Design review of the part built by this model. Coordinates are the model's own, in mm. Face numbers are marked on the shaded views. A direction names the side the tool comes from. Coordinates: 2 decimals unless noted, no trailing zeros. Write each loop counter-clockwise with the first axis right and the second up, starting at its lowest first coordinate (ties: lowest second). Pieces come first, ordered by that corner, then holes.
Q1. Add section C-C, the plane x = 40. Give the boundary of the cut face in (y, z).
Q2. Add section A-A, the plane y = 24. Give the boundary of the cut face in (x, z) (3 decimals), plus the area to 3 significant figures.
Q3. To check wall thickness, follow probe 1 along X at (y, z) = (157, -73); probe 2 along Z at (x, y) = (-6.5, 123.5); probe 3 along Z at (x, y) = (54, 81.5). State the ranges of each line that lie inside material, in increasing order.
Q4. Machinability: for the marked faces 4, 5 and 6, which of the approach directions +Z, -Z, +X, -X, +Y, -Y give a long, thin tool a straight path to every point of the face, cutting with its end or side? Answer none if there is none.
Q5. Clearance check with flat-ended pins moving along their axes: pin 1 Ø9.5 at (y, z) = (230, -51) entering from -X (3 decimals); pin 2 Ø2 at (x, z) = (218, 40.5) entering from +Y; pin 3 Ø15 at (x, y) = (-10, 100) entering from -Z. State where each tip first meets the part, or that it passes through.
Q6. Add section B-B, the plane z = -71. Give the boundary of the cut face in (x, y) (3 decimals).
Q7. Add section D-D, the plane y = 218. Give the boundary of the cut face in (x, z) (3 decimals).
Q8. The part is to be moulded in two halves that separate along Y. For the marked faces 1, 2 and 3, say which applies: +Y half, -Y half, draft (parallel to the pull), parting line (faces both ways), or undercut.
Autodesk Inventor part; units mm, degrees
ref_plane "Work Plane1" through (0, 104.775, 0) normal (0, 1, 0) x (-1, 0, 0)
ref_plane "Work Plane2" through (295.275, 0, -196.85) normal (-1, 0, 0) x (0, 0, 1)
ref_plane "YZ Plane" through (0, 0, 0) normal (1, 0, 0) x (0, 1, 0)
sketch "Sketch1" plane through (0, 0, 0) normal (1, 0, 0) x (0, 1, 0)
  line L0 (0, 120.65) -> (184.15, 120.65)
  line L1 (184.15, 120.65) -> (184.15, -120.65)
  line L2 (184.15, -120.65) -> (0, -120.65)
  line L3 (0, -120.65) -> (0, 120.65)
  point P0 (0, 0)
  point P1 (0, 0)
  dimension "d0" = 184.15
  dimension "d1" = 241.3
extrude "Extrusion1" add sketch "Sketch1" along normal blind 295.275
sketch "Sketch2" plane through (0, 0, 0) normal (-1, 0, 0) x (0, 0, 1)
  line L0 (120.65, 0) -> (120.65, 184.15) construction
  line L1 (120.65, 184.15) -> (-120.65, 184.15) construction
  line L2 (-120.65, 184.15) -> (-120.65, 0) construction
  line L3 (-120.65, 0) -> (120.65, 0) construction
  line L4 (-107.95, 171.45) -> (107.95, 171.45)
  line L5 (107.95, 171.45) -> (107.95, 12.7)
  line L6 (107.95, 12.7) -> (-107.95, 12.7)
  line L7 (-107.95, 12.7) -> (-107.95, 171.45)
  point P0 (0, 0)
  dimension "d4" = 12.7
extrude "Extrusion2" add sketch "Sketch2" along normal blind 19.05
ref_plane "Work Plane1" through (0, 104.775, 0) normal (0, 1, 0) x (-1, 0, 0)
sketch "Sketch3" plane through (0, 104.775, 0) normal (0, 1, 0) x (-1, 0, 0)
  line L0 (0, 120.65) -> (0, -120.65) construction
  line L1 (133.2378, 0) -> (-22.2063, 0) construction
  line L2 (0, 0) -> (19.05, 0)
  arc A0 (19.05, 0) -> (95.25, 76.2) centre (19.05, 76.2) ccw
  dimension "d8" = 19.05
  dimension "d22" = 76.2
sketch "Sketch4" plane through (0, 0, 0) normal (-1, 0, 0) x (0, 0, 1)
  circle A0 centre (0, 104.775) radius 9.525
  point P0 (0, 0)
  dimension "d9" = 19.05
sweep "Sweep1" add profiles "Sketch4" path "Sketch3"
sketch "Sketch5" plane through (0, 0, 0) normal (0, 1, 0) x (-1, 0, 0)
  line L0 (-295.275, 120.65) -> (-295.275, -120.65) construction
  line L1 (-295.275, 57.15) -> (-666.75, 57.15)
  line L2 (-666.75, 57.15) -> (-666.75, -196.85)
  line L3 (-666.75, -196.85) -> (-295.275, -196.85)
  line L4 (-295.275, -196.85) -> (-295.275, 57.15)
  line L5 (0, -120.65) -> (0, 120.65) construction
  point P0 (0, 0)
  dimension "d12" = 666.75
  dimension "d13" = 76.2
  dimension "d14" = 254
extrude "Extrusion3" add sketch "Sketch5" along normal blind 355.6
sketch "Sketch6" plane through (0, 0, 0) normal (0, 1, 0) x (-1, 0, 0)
  line L0 (-168.275, -63.5) -> (-295.275, -63.5)
  line L1 (-295.275, -63.5) -> (-295.275, -44.45)
  line L2 (-295.275, -44.45) -> (-168.275, -44.45)
  line L3 (-168.275, -44.45) -> (-168.275, -63.5)
  line L4 (-295.275, -196.85) -> (-295.275, 57.15) construction
  line L5 (0, -120.65) -> (-295.275, -120.65) construction
  point P0 (0, 0)
  dimension "d17" = 127
  dimension "d18" = 19.05
  dimension "d19" = 57.15
extrude "Extrusion4" add sketch "Sketch6" along normal blind 247.65
ref_plane "Work Plane2" through (295.275, 0, -196.85) normal (-1, 0, 0) x (0, 0, 1)
split_face "Split1"
properties part number "Welder" material "Steel"
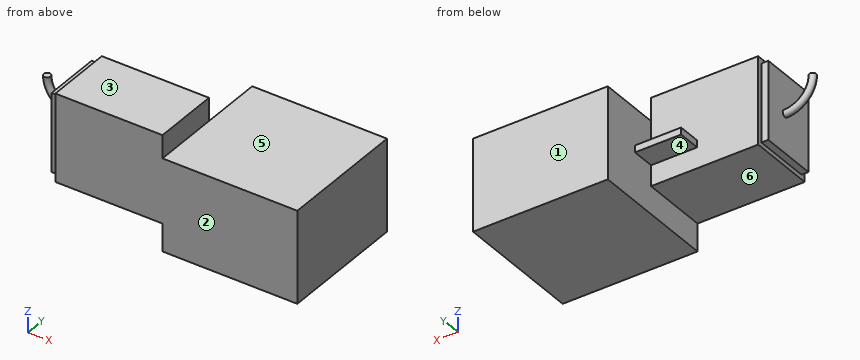
Here are the results:
1. outline: (0, -120.65) - (184.15, -120.65) - (184.15, 120.65) - (0, 120.65) - close
2. outline: (-19.05, -107.95) - (0, -107.95) - (0, -120.65) - (295.275, -120.65) - (295.275, -196.85) - (666.75, -196.85) - (666.75, 57.15) - (295.275, 57.15) - (295.275, 120.65) - (0, 120.65) - (0, 107.95) - (-19.05, 107.95) - close
2. area: 170,000 mm2
3. probe 1: x = -19.05 to 666.75
3. probe 2: z = -107.95 to 107.95
3. probe 3: z = -120.65 to 120.65
4. face 4: -Z, -X, +Y
4. face 5: +Z, +X, +Y, -Y
4. face 6: -Z, -X, +Y, -Y
5. pin 1: stops at x = 168.275
5. pin 2: stops at y = 184.15
5. pin 3: stops at z = -107.95
6. outline: (-19.05, 12.7) - (0, 12.7) - (0, 0) - (666.75, 0) - (666.75, 355.6) - (295.275, 355.6) - (295.275, 184.15) - (0, 184.15) - (0, 171.45) - (-19.05, 171.45) - close
7. outline: (168.275, -63.5) - (295.275, -63.5) - (295.275, -196.85) - (666.75, -196.85) - (666.75, 57.15) - (295.275, 57.15) - (295.275, -44.45) - (168.275, -44.45) - close
8. face 1: +Y half
8. face 2: -Y half
8. face 3: draft
